Geometry: final body of the model. Coordinates: model frame, mm. A direction names the side the tool comes from. Round coordinates to 2 decimals unless told otherwise and drop trailing zeros. Loops run counter-clockwise (first coordinate to the right, second up) from the corner with the lowest first, then second, coordinate; pieces in that order, holes last. Notation, with made-up numbers: M -7.5,10.25 L 19.5,10.25 A18 cw 19.5,19.25 Z; hole C 60,79.25 d9. An arc over 180 degrees is marked long. Answer as a JSON object with one key per item and string values.
from build123d import *

# Parameters (mm, degrees)
CUT_EXTRUDE1_DEPTH      = 236
CUT_EXTRUDE1_DEPTH_BACK = 258
SKETCH2_R               = 75
CUT_EXTRUDE2_DEPTH      = 17


with BuildPart() as part:
    # Sketch1 → Revolve1 (revolve)
    with BuildSketch(Plane.XY, mode=Mode.PRIVATE) as revolve1_sk:
        with BuildLine():
            Line((0, 0), (100, 0))
            Line((100, 0), (100, 210))
            Line((100, 210), (82.499679128, 210))
            ThreePointArc((82.499679128, 210), (50.072209241, 177.355662093), (17.5, 209.855581875))
            Line((17.5, 209.855581875), (0, 209.855581875))
            Line((0, 209.855581875), (0, 0))
        make_face()
    revolve(revolve1_sk.sketch.rotate(Axis((0, 0, 0), (1, 0, 0)), 90), axis=Axis((0, 0, 0), (1, 0, 0)))

    # Sketch2 → Cut-Extrude1 (cut, two sides: drawn at the far end of the back side and taken through both)
    with BuildSketch(Plane(origin=(100, 0, 0), x_dir=(0, 0, -1), z_dir=(1, 0, 0)).offset(-CUT_EXTRUDE1_DEPTH_BACK)):
        with Locations(Location((0, 0, 0), (0, 0, 180))):
            Circle(SKETCH2_R)
    extrude(amount=CUT_EXTRUDE1_DEPTH + CUT_EXTRUDE1_DEPTH_BACK, mode=Mode.SUBTRACT)

    # Sketch3 → Cut-Extrude2 (cut)
    with BuildSketch(Plane.ZY):
        with BuildLine():
            Line((20, 103.07764064), (53.626367642, 161.32021787))
            ThreePointArc((53.626367642, 161.32021787), (0, 170), (-53.626367642, 161.32021787))
            Line((-53.626367642, 161.32021787), (-20, 103.07764064))
            ThreePointArc((-20, 103.07764064), (0, 105), (20, 103.07764064))
        make_face()
        with BuildLine():
            Line((112.894222998, 127.101905625), (79.267855357, 68.859328396))
            ThreePointArc((79.267855357, 68.859328396), (90.932667397, 52.5), (99.267855357, 34.218312245))
            Line((99.267855357, 34.218312245), (166.52059064, 34.218312245))
            ThreePointArc((166.52059064, 34.218312245), (147.224318643, 85), (112.894222998, 127.101905625))
        make_face()
        with BuildLine():
            Line((166.52059064, -34.218312245), (99.267855357, -34.218312245))
            ThreePointArc((99.267855357, -34.218312245), (90.932667397, -52.5), (79.267855357, -68.859328396))
            Line((79.267855357, -68.859328396), (112.894222998, -127.101905625))
            ThreePointArc((112.894222998, -127.101905625), (147.224318643, -85), (166.52059064, -34.218312245))
        make_face()
        with BuildLine():
            Line((53.626367642, -161.32021787), (20, -103.07764064))
            ThreePointArc((20, -103.07764064), (0, -105), (-20, -103.07764064))
            Line((-20, -103.07764064), (-53.626367642, -161.32021787))
            ThreePointArc((-53.626367642, -161.32021787), (0, -170), (53.626367642, -161.32021787))
        make_face()
        with BuildLine():
            Line((-112.894222998, -127.101905625), (-79.267855357, -68.859328396))
            ThreePointArc((-79.267855357, -68.859328396), (-90.932667397, -52.5), (-99.267855357, -34.218312245))
            Line((-99.267855357, -34.218312245), (-166.52059064, -34.218312245))
            ThreePointArc((-166.52059064, -34.218312245), (-147.224318643, -85), (-112.894222998, -127.101905625))
        make_face()
        with BuildLine():
            Line((-166.52059064, 34.218312245), (-99.267855357, 34.218312245))
            ThreePointArc((-99.267855357, 34.218312245), (-90.932667397, 52.5), (-79.267855357, 68.859328396))
            Line((-79.267855357, 68.859328396), (-112.894222998, 127.101905625))
            ThreePointArc((-112.894222998, 127.101905625), (-147.224318643, 85), (-166.52059064, 34.218312245))
        make_face()
    cut_extrude2 = extrude(amount=-CUT_EXTRUDE2_DEPTH, mode=Mode.SUBTRACT)

    # Mirror1: Cut-Extrude2 across plane
    add(cut_extrude2.mirror(Plane(origin=(50, 0, 0), x_dir=(0, 0, 1), z_dir=(1, 0, 0))), mode=Mode.SUBTRACT)


solid = part.part
1) Section query C-C (x = 55.5). Return the cut outline in (y, z).
Results:
{"outline": "C 0,0 d355.65; hole C 0,0 d150"}
2) Pull-direction query (Z, two-part tool) for faces 4 (the flat face through (0, -3, 90)), 5 (the cylindrical face through (8.381, -84.338, -147.605)); classes: +Z half, -Z half, draft (parallel to the pull), parting line (faces both ways), or undercut.
Results:
{"face 4": "draft", "face 5": "undercut"}
3) Ray query, line 1 (Z direction, x = 16.5, y = -101); line 2 (Y direction, x = 87, z = -47.5); line 3 (Z direction, x = 91, y = 61.5). Return the intervals inside material, ascending.
Results:
{"line 1": "-183.95 to -136.74, -97.82 to 97.82, 136.74 to 183.95", "line 2": "-204.56 to -163.23, -150.71 to -58.04, 58.04 to 150.71, 163.23 to 204.56", "line 3": "-200.79 to -158.49, -85.1 to -42.93, 42.93 to 85.1, 158.49 to 200.79"}
4) Section query A-A (z = 0). Return the cut outline in (x, y).
Results:
{"outline": "M 0,-209.86 L 17.5,-209.86 A32.5 cw 82.5,-210 L 100,-210 L 100,-170 L 83,-170 L 83,-105 L 100,-105 L 100,-75 L 0,-75 L 0,-105 L 17,-105 L 17,-170 L 0,-170 Z; M 0,75 L 100,75 L 100,105 L 83,105 L 83,170 L 100,170 L 100,210 L 82.5,210 A32.5 cw 17.5,209.86 L 0,209.86 L 0,170 L 17,170 L 17,105 L 0,105 Z"}
5) Pin query (flat end, axial travel): P1, Ø5, axis at x = 95, z = 116.5, coming from the -Y side; P2, Ø20, axis at y = 141, z = -20, coming from the +X side; P3, Ø6, axis at x = 53, z = -104.5, coming from the +Y side; P4, Ø12, axis at y = -44.5, z = 51, coming from the -X side. Return the tip coordinate at first contact, or that it passes through.
Results:
{"P1": "y = -176.36", "P2": "x = 83", "P3": "y = 145.64", "P4": "through"}
6) Section query B-B (y = 0). Return the cut outline in (x, z), and give its area (3 significant figures).
Results:
{"outline": "M 0,-209.86 L 17.5,-209.86 A32.5 cw 82.5,-210 L 100,-210 L 100,-75 L 0,-75 Z; M 0,75 L 100,75 L 100,210 L 82.5,210 A32.5 cw 17.5,209.86 L 0,209.86 Z", "area": "23,700 mm2"}
7) Reachability of faces 1 (the flat face through (8.381, 131.791, 36.578)), 2 (the flat face through (91.619, 97.573, -95.846)), 3 (the cylindrical face through (49.3, 66.538, 34.608)) from +Z, -Z, +X, -X, +Y, -Y: full face, straight path, thin tool, end or side. Return the list, or none.
Results:
{"face 1": "-X", "face 2": "+X", "face 3": "+X, -X"}
